Work out the finished part from the listing and answer in its coordinate system (mm). Coordinates: 2 decimals unless noted, no trailing zeros. Write each loop counter-clockwise with the first axis right and the second up, starting at its lowest first coordinate (ties: lowest second). Pieces come first, ordered by that corner, then holes. Notation, with made-up numbers: (31.25, -40) - (83.25, -40) arc R22 cw to (83.25, -9) - close; hole circle Ø2 at (37.25, -27). An arc over 180 degrees is marked (long way). Use a Markdown table: item, result. Add a question column.
(1) Find the intervals of material crossed by line 1 (X direction, y = 0.1, z = 0); line 2 (Z direction, x = -56, y = 0.2); line 3 (Z direction, x = -45, y = 0.1), in increasing order. Write a range as from..to.
(2) The part is cut by section C-C, the plane y = 0.15. Give the vertices of the cut face in (x, z), then the cut area to 3 significant figures.
(3) The part is cut by section A-A, the plane x = -58.5. Give the vertices of the cut face in (y, z).
(4) The part is cut by section D-D, the plane x = -51. Give the vertices of the cut face in (y, z).
(5) The part is cut by section B-B, the plane z = 0. Give the vertices of the cut face in (x, y).
from build123d import *

# Parameters (mm, degrees)
EXTRUDE1_DEPTH = 0.254
EXTRUDE2_DEPTH = 1.254
SKETCH3_R      = 1.63
EXTRUDE3_DEPTH = 1.254


with BuildPart() as part:
    # Sketch1 → Extrude1 (new body)
    with BuildSketch(Plane(origin=(0, 0, 0), x_dir=(1, 0, 0), z_dir=(0, 1, 0))):
        Polygon((0, -11.5), (0, 11.5), (-12, 11.5), (-53.304347826, 2), (-55, 4), (-62, 4), (-62, -4), (-55, -4), (-53.304347826, -2), (-12, -11.5), align=None)
    extrude(amount=EXTRUDE1_DEPTH)

    # Sketch2 → Extrude2 (cut, through all)
    with BuildSketch(Plane(origin=(0, 0.254, 0), x_dir=(1, 0, 0), z_dir=(0, 1, 0))):
        with BuildLine():
            Line((-6, 4), (0, 4))
            Line((0, 4), (0, 8.5))
            Line((0, 8.5), (-6, 8.5))
            ThreePointArc((-6, 8.5), (-8.25, 6.25), (-6, 4))
        make_face()
        with BuildLine():
            Line((0, -8.5), (-6, -8.5))
            ThreePointArc((-6, -8.5), (-8.25, -6.25), (-6, -4))
            Line((-6, -4), (0, -4))
            Line((0, -4), (0, -8.5))
        make_face()
    extrude(amount=-EXTRUDE2_DEPTH, mode=Mode.SUBTRACT)

    # Sketch3 → Extrude3 (cut, through all)
    with BuildSketch(Plane(origin=(0, 0.254, 0), x_dir=(1, 0, 0), z_dir=(0, 1, 0))):
        with Locations(Location((-58.5, 0, 0), (0, 0, 270))):  # turned: the seam where the file's is
            Circle(SKETCH3_R)
    extrude(amount=-EXTRUDE3_DEPTH, mode=Mode.SUBTRACT)


solid = part.part
Model answer:
| question | item | result |
|---|---|---|
| 1 | line 1 | -62..-60.13, -56.87..0 |
| 1 | line 2 | -4..4 |
| 1 | line 3 | -3.91..3.91 |
| 2 | outline | (-62, -4) - (-55, -4) - (-53.3, -2) - (-12, -11.5) - (0, -11.5) - (0, -8.5) - (-6, -8.5) arc R2.25 cw to (-6, -4) - (0, -4) - (0, 4) - (-6, 4) arc R2.25 cw to (-6, 8.5) - (0, 8.5) - (0, 11.5) - (-12, 11.5) - (-53.3, 2) - (-55, 4) - (-62, 4) - close; hole circle Ø3.26 at (-58.5, 0) |
| 2 | area | 822 mm^2 |
| 3 | outline | (0, -4) - (0.25, -4) - (0.25, -1.63) - (0, -1.63) - close; (0, 1.63) - (0.25, 1.63) - (0.25, 4) - (0, 4) - close |
| 4 | outline | (0, -2.53) - (0.25, -2.53) - (0.25, 2.53) - (0, 2.53) - close |
| 5 | outline | (-62, 0) - (-60.13, 0) - (-60.13, 0.25) - (-62, 0.25) - close; (-56.87, 0) - (0, 0) - (0, 0.25) - (-56.87, 0.25) - close |
